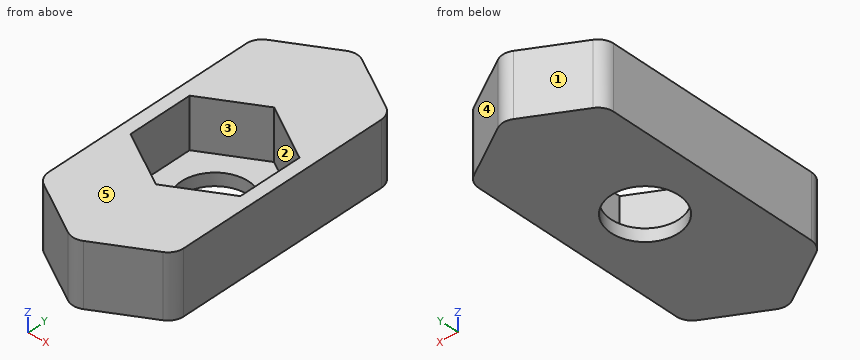
from build123d import *

# Parameters (mm, degrees)
F0_R     = 2.15
F1_DEPTH = 4
F2_DEPTH = 3.2
F3_R     = 1


with BuildPart() as f1:
    # F0 (on Top) → F1 (new body)
    with BuildSketch(Plane.XY):
        Polygon((4.3, -7.332348), (4.3, 7.332348), (0, 9.814955), (-4.3, 7.332348), (-4.3, -7.332348), (0, -9.814955), align=None)
        Polygon((0, 4.041452), (3.5, 2.020726), (3.5, -2.020726), (0, -4.041452), (-3.5, -2.020726), (-3.5, 2.020726), align=None, mode=Mode.SUBTRACT)
        Polygon((3.5, -2.020726), (3.5, 2.020726), (0, 4.041452), (-3.5, 2.020726), (-3.5, -2.020726), (0, -4.041452), align=None)
        Circle(F0_R, mode=Mode.SUBTRACT)
    extrude(amount=-F1_DEPTH)

    # F0 (on Top) → F2 (cut)
    with BuildSketch(Plane.XY):
        Polygon((3.5, -2.020726), (3.5, 2.020726), (0, 4.041452), (-3.5, 2.020726), (-3.5, -2.020726), (0, -4.041452), align=None)
        Circle(F0_R, mode=Mode.SUBTRACT)
    extrude(amount=-F2_DEPTH, mode=Mode.SUBTRACT)

    # F3
    f3_edges = [f1.edges().sort_by_distance(p)[0] for p in [
        (-4.3, 7.332348, -2),
        (0, 9.814955, -2),
        (4.3, 7.332348, -2),
        (4.3, -7.332348, -2),
        (0, -9.814955, -2),
        (-4.3, -7.332348, -2),
    ]]
    fillet(f3_edges, radius=F3_R)


solid = f1.part
Check sheet for the modelled part. Datum: model origin and axes. Units: mm. Face numbers are marked on the shaded views. A direction names the side the tool comes from. Round coordinates to 2 decimals unless told otherwise and drop trailing zeros. Loops run counter-clockwise (first coordinate to the right, second up) from the corner with the lowest first, then second, coordinate; pieces in that order, holes last.
1. Sectioned sample at D-D on x = -2.5. Record the boundary of the cut face in (y, z).
2. Set-up check for the marked faces 1 and 2: record each of +Z, -Z, +X, -X, +Y, -Y from which the full face is reachable in a straight line by a thin tool's end or side.
3. Sectioned sample at A-A on z = -2.75. Record the boundary of the cut face in (x, y) (3 decimals).
4. Sectioned sample at B-B on y = 0. Record the boundary of the cut face in (x, z), and give its area (3 significant figures).
5. Gauge pin test, flat end, axial feed: pin 1 Ø2 at (x, z) = (-2, -3) entering from -Y. Record the tip position at first contact, or that the pin passes through.
6. Sectioned sample at C-C on x = 1.5. Record the boundary of the cut face in (y, z), and give its area (3 significant figures).
7. Mould release check, pull along X, two halves, no side actions. Record for the marked faces 3, 4 and 5: released by +X, released by -X, zero draft, split by the parting line, or undercut.
8. Scan lines: probe 1 along Y at (x, z) = (0, -3.8); probe 2 along X at (y, z) = (1, -3.1); probe 3 along Y at (x, z) = (-2, -1.25). Record each from-to range of solid material in increasing order.
Recorded:
1. outline: (-8.37, -4) - (8.37, -4) - (8.37, 0) - (2.6, 0) - (2.6, -3.2) - (-2.6, -3.2) - (-2.6, 0) - (-8.37, 0) - close
2. face 1: +Z, -Z, -X, +Y
2. face 2: +Z
3. outline: (-4.3, -6.755) arc R1 ccw to (-3.8, -7.621) - (-0.5, -9.526) arc R1 ccw to (0.5, -9.526) - (3.8, -7.621) arc R1 ccw to (4.3, -6.755) - (4.3, 6.755) arc R1 ccw to (3.8, 7.621) - (0.5, 9.526) arc R1 ccw to (-0.5, 9.526) - (-3.8, 7.621) arc R1 ccw to (-4.3, 6.755) - close; hole (-3.5, -2.021) - (0, -4.041) - (3.5, -2.021) - (3.5, 2.021) - (0, 4.041) - (-3.5, 2.021) - close
4. outline: (-4.3, -4) - (-2.15, -4) - (-2.15, -3.2) - (-3.5, -3.2) - (-3.5, 0) - (-4.3, 0) - close; (2.15, -4) - (4.3, -4) - (4.3, 0) - (3.5, 0) - (3.5, -3.2) - (2.15, -3.2) - close
4. area: 8.56 mm2
5. pin 1: stops at y = -9.24
6. outline: (-8.95, -4) - (-1.54, -4) - (-1.54, -3.2) - (-3.18, -3.2) - (-3.18, 0) - (-8.95, 0) - close; (1.54, -4) - (8.95, -4) - (8.95, 0) - (3.18, 0) - (3.18, -3.2) - (1.54, -3.2) - close
6. area: 48.8 mm2
7. face 3: undercut
7. face 4: released by +X
7. face 5: zero draft
8. probe 1: y = -9.66 to -2.15, 2.15 to 9.66
8. probe 2: x = -4.3 to -3.5, 3.5 to 4.3
8. probe 3: y = -8.66 to -2.89, 2.89 to 8.66
